Autodesk Inventor part; units mm, degrees
ref_plane "YZ Plane" through (0, 0, 0) normal (1, 0, 0) x (0, 1, 0)
ref_plane "XZ Plane" through (0, 0, 0) normal (0, 1, 0) x (-1, 0, 0)
ref_plane "XY Plane" through (0, 0, 0) normal (0, 0, 1) x (1, 0, 0)
sketch "스케치1" plane through (0, 0, 0) normal (0, 0, 1) x (1, 0, 0)
  line L0 (0, 0) -> (22.5, 0)
  line L1 (22.5, 0) -> (22.5, 12.3)
  line L2 (0, 12.3) -> (0, 0)
  line L3 (-5, -3) -> (27.5, -3)
  line L4 (27.5, -3) -> (27.5, 12.3)
  line L5 (27.5, 12.3) -> (22.5, 12.3)
  line L6 (-5, 12.3) -> (-5, -3)
  line L7 (0, 12.3) -> (-5, 12.3)
  dimension "d0" = 22.5
  dimension "d1" = 12.3
  dimension "d2" = 32.5
extrude "돌출1" add sketch "스케치1" against normal blind 10
hole "구멍1" at (25, 6, 0) direction (0, 0, -1) diameter 1.5 depth 10 tip angle 118
hole "구멍2" at (-2.5, 6, 0) direction (0, 0, -1) diameter 1.5 depth 10 tip angle 118
sketch "스케치3" plane through (-5, -3, 0) normal (0, -1, 0) x (1, 0, 0)
  line L0 (32.5, 0) -> (32.5, -10)
  line L1 (0, 0) -> (32.5, 0)
  line L2 (32.5, 0) -> (32.5, -3)
  line L3 (32.5, -3) -> (0, -3)
  line L4 (0, -3) -> (0, 0)
  point P0 (5, 0)
  point P1 (32.5, -13)
  dimension "d34" = 3
extrude "돌출3" add sketch "스케치3" along normal blind 12
sketch "스케치4" plane through (27.5, -3, -3) normal (0, 0, -1) x (-1, 0, 0)
  line L0 (27.5, -3) -> (5, -3) construction
  line L1 (27.5, -1.375) -> (5, -1.375)
  line L2 (5, -4.625) -> (27.5, -4.625)
  arc A0 (27.5, -4.625) -> (27.5, -1.375) centre (27.5, -3) ccw
  arc A1 (5, -1.375) -> (5, -4.625) centre (5, -3) ccw
  point P0 (27.5, 3)
  point P1 (16.25, -3)
  dimension "d38" = 22.5
  dimension "d39" = 3.25
extrude "돌출4" cut sketch "스케치4" against normal through all
sketch "스케치5" plane through (0, 0, -10) normal (0, 0, -1) x (-1, 0, 0)
  arc A0 (-22.5, -4.375) -> (-22.5, -7.625) centre (-22.5, -6) ccw
  line L0 (-22.5, -4.375) -> (0, -4.375)
  line L1 (0, -7.625) -> (-22.5, -7.625)
  arc A1 (0, -7.625) -> (0, -4.375) centre (0, -6) ccw
  line L2 (-22.5, -6) -> (0, -6) construction
  line L3 (-22.5, -9.75) -> (0, -9.75)
  line L4 (0, -2.25) -> (-22.5, -2.25)
  arc A2 (-22.5, -2.25) -> (-22.5, -9.75) centre (-22.5, -6) ccw
  arc A3 (0, -9.75) -> (0, -2.25) centre (0, -6) ccw
  point P0 (0, 0)
  point P1 (-11.25, -6)
  dimension "d40" = 7.5
extrude "돌출5" cut sketch "스케치5" against normal up to surface (7 mm away) contours L0 A1 L1 A0 | A2 L4 A3 L3
chamfer "모따기1" distance 5 angle 45 2 edges at (-3.625, -3, -3) (26.125, -3, -3)
properties part number "servolock1"
Build history of the part. All positions in model axes, mm. A direction names the side the tool comes from. Give positions to 0.01 mm unless a question says otherwise; leave off trailing zeros. Loops run counter-clockwise (first coordinate to the right, second up) from the corner with the lowest first, then second, coordinate; pieces in that order, holes last. Notation, with made-up numbers: (-27.5, -1) -> (-3.5, -1) arc R13 ccw to (-3.5, 24) -> close; hole circle Ø4 at (-32, 33.25). An arc over 180 degrees is marked (long way). One line per question, with ' | ' between items.
Q1. Cut at D-D, the plane z = -1.5. Write the cut outline in (x, y) (3 decimals), plus the area to 3 significant figures.
Filled sheet:
outline: (-5, -15) -> (27.5, -15) -> (27.5, 12.3) -> (22.5, 12.3) -> (22.5, 0) -> (0, 0) -> (0, 12.3) -> (-5, 12.3) -> close; hole circle Ø1.5 at (-2.5, 6); hole (0, -7.625) -> (22.5, -7.625) arc R1.625 ccw to (22.5, -4.375) -> (0, -4.375) arc R1.625 ccw to start; hole circle Ø1.5 at (25, 6) | area: 526 mm²
Q2. Cut at A-A, the plane x = 1. Write the cut outline in (y, z) (3 decimals).
Filled sheet:
outline: (-15, -3) -> (-7.625, -3) -> (-7.625, 0) -> (-15, 0) -> close; (-4.375, -3) -> (-2.25, -3) -> (-2.25, -10) -> (0, -10) -> (0, 0) -> (-4.375, 0) -> close
Q3. Tool access for faces 1 (the flat face through (0, 6, -5)), 2 (the flat face through (11, -7.625, -2)), 3 (the flat face through (11, -2.25, -7)), 4 (the flat face through (27.5, 2, -4)), 5 (the flat face through (-4, -3, -9)): list every direction of +Z, -Z, +X, -X, +Y, -Y with a clear straight run to the whole face (end or side of a thin tool).
Filled sheet:
face 1: +Z, -Z, +Y | face 2: +Z, -Z | face 3: -Z, -Y | face 4: +Z, -Z, +X, +Y, -Y | face 5: -Z, +X, -X, -Y
Q4. Drop flat-ended pins along their axis: pin 1 (1.7 mm diameter, centred on x = 25, y = 6, fed in from +Z); pin 2 (3.5 mm diameter, centred on x = 10, z = -1.5, fed in from +Y); pin 3 (1 mm diameter, centred on x = 23, y = -9, fed in from -Z); pin 4 (1 mm diameter, centred on x = -3, z = -9, fed in from -Y). Give the stop position or say it passes through.
Filled sheet:
pin 1: stops at z = 0 | pin 2: stops at y = 0 | pin 3: stops at z = -3 | pin 4: stops at y = -3
Q5. Cut at C-C, the plane y = -6. Write the cut outline in (x, z) (3 decimals).
Filled sheet:
outline: (-5, -5) -> (-3.75, -5) -> (-3.75, -3) -> (-1.625, -3) -> (-1.625, 0) -> (-5, 0) -> close; (24.125, -3) -> (26.25, -3) -> (26.25, -5) -> (27.5, -5) -> (27.5, 0) -> (24.125, 0) -> close
Q6. Pull direction Y, two halves, no side cores. Call faces 6 (the cylindrical face through (24.125, -5.964, -1.521)), 7 (the flat face through (25, 12.3, -5)), 8 (the flat face through (22.5, 6, -5)): pulls with the +Y half, pulls with the -Y half, needs draft (parallel to the pull), parting line crosses it, or undercut.
Filled sheet:
face 6: undercut | face 7: pulls with the +Y half | face 8: needs draft
Q7. Cut at B-B, the plane y = 6. Write the cut outline in (x, z).
Filled sheet:
outline: (-5, -10) -> (-3.25, -10) -> (-3.25, 0) -> (-5, 0) -> close; (-1.75, -10) -> (0, -10) -> (0, 0) -> (-1.75, 0) -> close; (22.5, -10) -> (24.25, -10) -> (24.25, 0) -> (22.5, 0) -> close; (25.75, -10) -> (27.5, -10) -> (27.5, 0) -> (25.75, 0) -> close
Q8. Drill centre lines: line 1 along X through (y, z) = (9.25, -4); line 2 along Y through (x, z) = (16, -1.25) (3 decimals); line 3 along X through (y, z) = (6, -6.5). Where is each one in solid material? Low to high. Write a range as [from, to].
Filled sheet:
line 1: x = [-5, 0], [22.5, 27.5] | line 2: y = [-15, -7.625], [-4.375, 0] | line 3: x = [-5, -3.25], [-1.75, 0], [22.5, 24.25], [25.75, 27.5]
